Input: part model. Units: mm. Frame: model coordinates. Face numbers are marked on the shaded views. A direction names the side the tool comes from. Give positions to 0.01 mm unless a question says otherwise; leave off trailing zeros. Loops run counter-clockwise (first coordinate to the right, second up) from the corner with the lowest first, then second, coordinate; pieces in that order, holes last. Notation, with made-up numbers: (-29, 35.25) - (3, 35.25) arc R23 cw to (3, 62.25) - close; hole circle Ø11 at (78.25, 89). An arc over 180 degrees is marked (long way). One line per question, with ' | ' between items. Start each with the question number.
from build123d import *

# Parameters (mm, degrees)
SKETCH1_W           = 90.678
SKETCH1_H           = 88.9
SKETCH1_R           = 1.27
BOSS_EXTRUDE1_DEPTH = 10
SKETCH2_W           = 10
SKETCH2_H           = 88.9
BOSS_EXTRUDE2_DEPTH = 30
SKETCH5_W           = 10
SKETCH5_H           = 40
CUT_EXTRUDE1_DEPTH  = 10
SKETCH7_W           = 60
SKETCH7_H           = 88.9
BOSS_EXTRUDE3_DEPTH = 10
SKETCH8_R           = 2.5
CUT_EXTRUDE2_DEPTH  = 10


with BuildPart() as part:
    # Sketch1 → Boss-Extrude1 (new body)
    with BuildSketch(Plane.XY):
        with Locations((45.339, 44.45)):
            Rectangle(SKETCH1_W, SKETCH1_H)
        with Locations((2.921, 3.175)):
            Circle(SKETCH1_R, mode=Mode.SUBTRACT)
        with Locations((3.048, 85.979)):
            Circle(SKETCH1_R, mode=Mode.SUBTRACT)
        with Locations((87.884, 2.667)):
            Circle(SKETCH1_R, mode=Mode.SUBTRACT)
        with Locations((88.138, 86.36)):
            Circle(SKETCH1_R, mode=Mode.SUBTRACT)
    extrude(amount=BOSS_EXTRUDE1_DEPTH)

    # Sketch2 → Boss-Extrude2 (add)
    with BuildSketch(Plane.ZY):
        with Locations((5, 44.45)):
            Rectangle(SKETCH2_W, SKETCH2_H)
    extrude(amount=BOSS_EXTRUDE2_DEPTH)

    # Sketch5 → Cut-Extrude1 (cut)
    with BuildSketch(Plane.XY.offset(10)):
        with Locations((-17, 44.45)):
            Rectangle(SKETCH5_W, SKETCH5_H)
    extrude(amount=-CUT_EXTRUDE1_DEPTH, mode=Mode.SUBTRACT)

    # Sketch7 → Boss-Extrude3 (add)
    with BuildSketch(Plane.ZY.offset(30)):
        with Locations((-20, 44.45)):
            Rectangle(SKETCH7_W, SKETCH7_H)
    extrude(amount=BOSS_EXTRUDE3_DEPTH)

    # Sketch8 → Cut-Extrude2 (cut)
    with BuildSketch(Plane.ZY.offset(40)):
        with Locations((-10, 68.9)):
            Circle(SKETCH8_R)
        with Locations(Location((-10, 20, 0), (0, 0, 180))):
            Circle(SKETCH8_R)
        with Locations((-30, 20)):
            Circle(SKETCH8_R)
        with Locations(Location((-30, 68.9, 0), (0, 0, 180))):
            Circle(SKETCH8_R)
    extrude(amount=-CUT_EXTRUDE2_DEPTH, mode=Mode.SUBTRACT)


solid = part.part
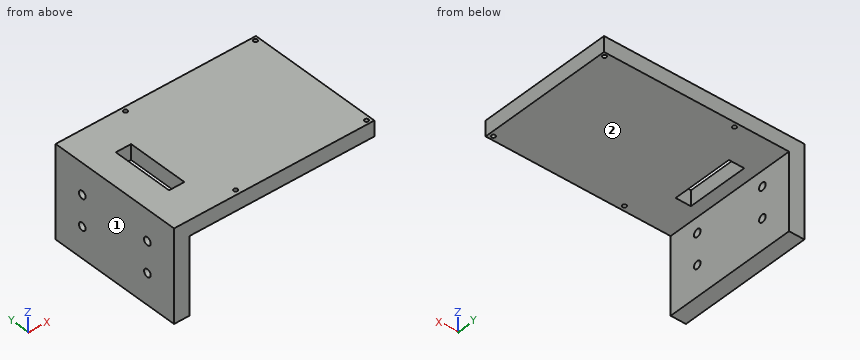
Q1. Access query for the marked faces 1 and 2. Directions: +Z, -Z, +X, -X, +Y, -Y. A direction counts if a zero-diameter tool reaches every point of the face in a straight line with its end or side. Return the directions, or none.
Q2. Section B-B, the plane y = 68.9. Output: boundary loops of the cut face in (x, z), plus the area to 3 significant figures.
Q3. First-contact query: pin 1 (3 mm diameter, centred on x = 2.921, y = 3.175, fed in from +Z); pin 2 (12 mm diameter, centred on x = -8, y = 32.5, fed in from -Z); pin 3 (3 mm diameter, centred on y = 28, z = -28.5, fed in from +X). Flat tips, straight axial feed; report the tip coordinate or a pass-through.
Q4. Section A-A, the plane x = -14. Output: boundary loops of the cut face in (y, z).
Q5. Line query: L1, parallel to Y at x = -34, z = -10; L2, parallel to Y at x = -13.5, z = 1.5; L3, parallel to X at y = 29.5, z = -21. Output: solid intervals per line, ascending. Write a range as from..to.
Q6. Section D-D, the plane y = 52.5. Output: boundary loops of the cut face in (x, z), plus the area to 3 significant figures.
Q7. Section C-C, the plane z = -10. Output: boundary loops of the cut face in (x, y), plus the area to 3 significant figures.
Solved:
1) face 1: +Z, -Z, -X, +Y, -Y | face 2: -Z, +X, +Y, -Y
2) outline: (-40, -50) - (-30, -50) - (-30, -32.5) - (-40, -32.5) - close; (-40, -27.5) - (-30, -27.5) - (-30, -12.5) - (-40, -12.5) - close; (-40, -7.5) - (-30, -7.5) - (-30, 0) - (90.68, 0) - (90.68, 10) - (-40, 10) - close | area: 1,710 mm²
3) pin 1: stops at z = 10 | pin 2: stops at z = 0 | pin 3: stops at x = -30
4) outline: (0, 0) - (24.45, 0) - (24.45, 10) - (0, 10) - close; (64.45, 0) - (88.9, 0) - (88.9, 10) - (64.45, 10) - close
5) L1: y = 0..17.5, 22.5..66.4, 71.4..88.9 | L2: y = 0..24.45, 64.45..88.9 | L3: x = -40..-30
6) outline: (-40, -50) - (-30, -50) - (-30, 0) - (-22, 0) - (-22, 10) - (-40, 10) - close; (-12, 0) - (90.68, 0) - (90.68, 10) - (-12, 10) - close | area: 1,710 mm²
7) outline: (-40, 0) - (-30, 0) - (-30, 17.5) - (-40, 17.5) - close; (-40, 22.5) - (-30, 22.5) - (-30, 66.4) - (-40, 66.4) - close; (-40, 71.4) - (-30, 71.4) - (-30, 88.9) - (-40, 88.9) - close | area: 789 mm²
